```python
from build123d import *

# Parameters (mm, degrees)
SKETCH1_W            = 40
SKETCH1_H            = 40
BOSS_EXTRUDE1_DEPTH  = 40
SKETCH2_W            = 20
SKETCH2_H            = 20
CUT_EXTRUDE1_DEPTH   = 40
CUT_EXTRUDE2_DEPTH   = 40
CUT_EXTRUDE6_DEPTH   = 40
CUT_EXTRUDE7_DEPTH   = 19.999
SKETCH7_W            = 19.998
SKETCH7_H            = 19.999
CUT_EXTRUDE8_DEPTH   = 19.999
SKETCH8_W            = 19.999
SKETCH8_H            = 19.999
CUT_EXTRUDE9_DEPTH   = 19.999
SKETCH11_W           = 28.28144282
SKETCH11_H           = 19.999
BOSS_EXTRUDE9_DEPTH  = 0.0009
BOSS_EXTRUDE10_DEPTH = 20
SKETCH14_W           = 57
SKETCH14_H           = 20
CUT_EXTRUDE11_DEPTH  = 20


with BuildPart() as part:
    # Sketch1 → Boss-Extrude1 (new body)
    with BuildSketch(Plane.XY):
        with Locations((20, 20)):
            Rectangle(SKETCH1_W, SKETCH1_H)
    extrude(amount=BOSS_EXTRUDE1_DEPTH)

    # Sketch2 → Cut-Extrude1 (cut)
    with BuildSketch(Plane.XY.offset(40)):
        with Locations((10, 30)):
            Rectangle(SKETCH2_W, SKETCH2_H)
    extrude(amount=-CUT_EXTRUDE1_DEPTH, mode=Mode.SUBTRACT)

    # Sketch3 → Cut-Extrude2 (cut)
    with BuildSketch(Plane.ZY.offset(-20)):
        Polygon((0, 20), (40, 40), (0, 40), align=None)
    extrude(amount=-CUT_EXTRUDE2_DEPTH, mode=Mode.SUBTRACT)

    # Sketch4 → Cut-Extrude6 (cut)
    with BuildSketch(Plane(origin=(0, 0, 0), x_dir=(1, 0, 0), z_dir=(0, 1, 0))):
        Polygon((0, 0), (20, -20), (20, -40), (0, -40), align=None)
    extrude(amount=CUT_EXTRUDE6_DEPTH, mode=Mode.SUBTRACT)

    # Sketch6 → Cut-Extrude7 (cut)
    with BuildSketch(Plane(origin=(0, 0, 0), x_dir=(-1, 0, 0), z_dir=(0, -1, 0))):
        Polygon((-20.001, -39.9999), (-39.999, -39.9999), (-20.001, -20.0019), align=None)
    extrude(amount=-CUT_EXTRUDE7_DEPTH, mode=Mode.SUBTRACT)

    # Sketch7 → Cut-Extrude8 (cut)
    with BuildSketch(Plane(origin=(20.001, 0, 0), x_dir=(0, 0, -1), z_dir=(1, 0, 0))):
        with Locations((-30.0009, 9.9995)):
            Rectangle(SKETCH7_W, SKETCH7_H)
    extrude(amount=-CUT_EXTRUDE8_DEPTH, mode=Mode.SUBTRACT)

    # Sketch8 → Cut-Extrude9 (cut)
    with BuildSketch(Plane(origin=(0, 0, 39.9999), x_dir=(-1, 0, 0), z_dir=(0, 0, -1))):
        with Locations((-29.9995, 9.9995)):
            Rectangle(SKETCH8_W, SKETCH8_H)
    extrude(amount=-CUT_EXTRUDE9_DEPTH, mode=Mode.SUBTRACT)

    # Sketch11 → Boss-Extrude9 (add)
    with BuildSketch(Plane(origin=(-0.00045, 0, 0.00045), x_dir=(0.707106781, 0, 0.707106781), z_dir=(-0.707106781, 0, 0.707106781))):
        with Locations((42.427043267, 9.9995)):
            Rectangle(SKETCH11_W, SKETCH11_H)
    extrude(amount=BOSS_EXTRUDE9_DEPTH)

    # Sketch13 → Boss-Extrude10 (add)
    with BuildSketch(Plane(origin=(0, 0, 0), x_dir=(-1, 0, 0), z_dir=(0, -1, 0))):
        Polygon((-20.001, -20.0019), (-20.000363604, -20.002536396), (-20, -20.0019), align=None)
    extrude(amount=-BOSS_EXTRUDE10_DEPTH)

    # Sketch14 → Cut-Extrude11 (cut)
    with BuildSketch(Plane(origin=(0, 0, 0), x_dir=(0.707106781, 0, 0.707106781), z_dir=(-0.707106781, 0, 0.707106781))):
        with Locations((28.5, 10)):
            Rectangle(SKETCH14_W, SKETCH14_H)
    extrude(amount=CUT_EXTRUDE11_DEPTH, mode=Mode.SUBTRACT)


solid = part.part
```
Here's how the part is built. I have some questions about the finished solid (model axes, mm). A direction names the side the tool comes from. Coordinates: 2 decimals unless noted, no trailing zeros. Order: outer loops, then holes, each group sorted by start corner. A loop starts at its lowest first (then second) coordinate and runs counter-clockwise, first axis right, second up. Notation, with made-up numbers: (50.5, 87) - (103.5, 87) arc R19 ccw to (103.5, 105) - close; hole circle Ø10 at (-7, 78). An arc over 180 degrees is marked (long way). One line per question, with ' | ' between items. Start each with the question number.
1. Which directions (+Z, -Z, +X, -X, +Y, -Y) give clear straight access to the entire face, cutting with the end or side of a thin tool? Please do faces 1 (the flat face through (26, 20, 34)), 2 (the flat face through (25, 0, 15)), 3 (the flat face through (20, 25, 29)).
2. Please list where these lines run through material, in increasing order: line 1 along X through (y, z) = (27, 21); line 2 along Z through (x, y) = (10, 4); line 3 along X through (y, z) = (16, 24). Write a range as [from, to].
3. I'm going to push flat-ended pins straight in: pin 1 Ø1.5 at (x, z) = (31, 18.5) entering from +Y (3 decimals); pin 2 Ø22 at (y, z) = (35, 24) entering from -X; pin 3 Ø10 at (x, z) = (11, 10.5) entering from +Y; pin 4 Ø12 at (x, y) = (7.5, 31) entering from +Z. Where does each tip first touch, or does it pass through?
4. If we section it at B-B (z = 36): Write out the boundary of the cut face in (x, y).
5. If we section it at A-A (x = 35): Write out the boundary of the cut face in (y, z).
6. If we section it at D-D (x = 14): Write out the boundary of the cut face in (y, z), and give its area (3 significant figures).
7. If we section it at C-C (y = 24): Write out the boundary of the cut face in (x, z), and give its area (3 significant figures).
Model answer:
1) face 1: +Z, -X, -Y | face 2: +Z, -Z, +X, -X, -Y | face 3: +Z, -Z, -X, +Y
2) line 1: x = [20, 40] | line 2: z = [0, 10] | line 3: x = [24, 40]
3) pin 1: stops at y = 29.625 | pin 2: stops at x = 20 | pin 3: stops at y = 20 | pin 4: passes through
4) outline: (20, 20) - (36, 20) - (36, 0) - (40, 0) - (40, 38) - (20, 38) - close
5) outline: (0, 0) - (20, 0) - (40, 40) - (20, 40) - (20, 35) - (0, 35) - close
6) outline: (0, 0) - (20, 0) - (20, 14) - (0, 14) - close | area: 280 mm²
7) outline: (20, 8) - (40, 8) - (40, 40) - (20, 40) - close | area: 640 mm²
